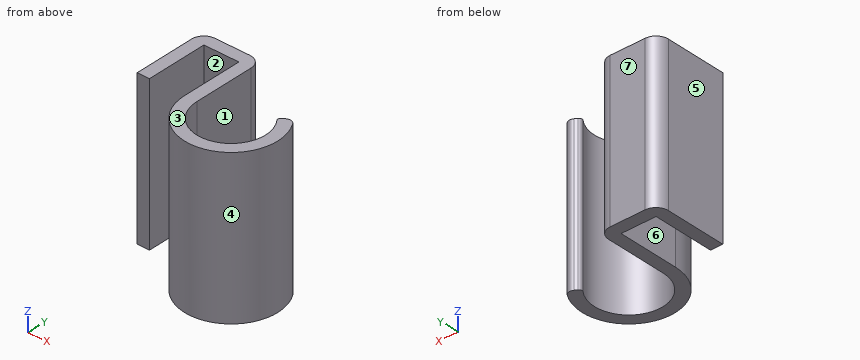
```python
from build123d import *

# Parameters (mm, degrees)
F1_DEPTH = 25
F2_R     = 2
F3_R     = 2
F4_R     = 1
F5_R     = 0.5


with BuildPart() as f1:
    # F0 (on Top) → F1 (new body)
    with BuildSketch(Plane.XY):
        with BuildLine():
            Line((7.7, 12), (-2, 12))
            Line((-2, 12), (-2, 0))
            Line((-2, 0), (0, 0))
            Line((0, 0), (0, 10))
            Line((0, 10), (5.7, 10))
            Line((5.7, 10), (5.7, 0))
            ThreePointArc((5.7, 0), (15.867507, -7.153175), (19.165239, 4.833112))
            Line((19.165239, 4.833112), (17.410544, 3.803082))
            ThreePointArc((17.410544, 3.803082), (15.342175, -5.214357), (7.7, 0))
            Line((7.7, 0), (7.7, 12))
        make_face()
    extrude(amount=F1_DEPTH)

    # F2
    f2_edges = [f1.edges().sort_by_distance(p)[0] for p in [
        (7.7, 12, 12.5),
    ]]
    fillet(f2_edges, radius=F2_R)

    # F3
    f3_edges = [f1.edges().sort_by_distance(p)[0] for p in [
        (-2, 12, 12.5),
    ]]
    fillet(f3_edges, radius=F3_R)

    # F4
    f4_edges = [f1.edges().sort_by_distance(p)[0] for p in [
        (19.165239, 4.833112, 12.5),
    ]]
    fillet(f4_edges, radius=F4_R)

    # F5
    f5_edges = [f1.edges().sort_by_distance(p)[0] for p in [
        (17.410544, 3.803082, 12.5),
    ]]
    fillet(f5_edges, radius=F5_R)


solid = f1.part
```
Here's how the part is built. I have some questions about the finished solid (model axes, mm). Face numbers are marked on the shaded views. A direction names the side the tool comes from. Coordinates: 2 decimals unless noted, no trailing zeros. Loops run counter-clockwise (first coordinate to the right, second up) from the corner with the lowest first, then second, coordinate; pieces in that order, holes last. Notation, with made-up numbers: (26, -24) - (36, -24) arc R13 cw to (36, -11) - close; hole circle Ø5 at (40.5, -25.75). An arc over 180 degrees is marked (long way). Return JSON: item names as keys, results as strings. Group by question number.
Item 1: If we section it at C-C on x = 13.3: Write out the boundary of the cut face in (y, z), and give its area (3 significant figures).
Item 2: If we section it at A-A on y = 6.25: Write out the boundary of the cut face in (x, z), and give its area (3 significant figures).
Item 3: On a 3-axis mill with a long thin cutter (end or side, diameter ignored), from which of +Z, -Z, +X, -X, +Y, -Y can I reach the whole of each face in a straight line? I mean the marked faces 1, 2 and 3. Say none if no direction works.
Item 4: We'd pull the mould along X, two halves only. Please class the marked faces 4, 5, 6 and 7: +X half, -X half, draft (parallel to the pull), parting line (faces both ways), or undercut.
Item 5: Will these pins go through, and if not, where does the flat tip stop? P1, Ø1.5, axis at x = 3, y = 7.5, coming from the -Z side; P2, Ø6, axis at y = -3.5, z = 16, coming from the -X side; P3, Ø1.6, axis at x = -0.5, z = 15.5, coming from the -Y side; P4, Ø1, axis at y = -3.5, z = 20, coming from the +X side.
Item 6: If we section it at B-B on z = 13.25: Write out the boundary of the cut face in (x, y).
Item 7: If we section it at D-D on x = 6.75: Write out the boundary of the cut face in (y, z).
Item 8: I need wall thicknesses on line 1 (X direction, y = 5.25, z = 10); line 2 (X direction, y = -0.25, z = 19.75); line 3 (Y direction, x = 17.75, z = 13.5). Which ranges of each line are inside material? Lowest first, please. Write a range as from..to.
Calculated:
{
 "1": {"outline": "(-7.6, 0) - (-5.6, 0) - (-5.6, 25) - (-7.6, 25) - close", "area": "50.0 mm^2"},
 "2": {"outline": "(-2, 0) - (0, 0) - (0, 25) - (-2, 25) - close; (5.7, 0) - (7.7, 0) - (7.7, 25) - (5.7, 25) - close", "area": "100 mm^2"},
 "3": {"face 1": "+Z, -Z, +Y", "face 2": "+Z, -Z, -Y", "face 3": "+Z, +X, -X, +Y, -Y"},
 "4": {"face 4": "parting line", "face 5": "-X half", "face 6": "undercut", "face 7": "draft"},
 "5": {"P1": "passes through", "P2": "stops at x = 5.72", "P3": "stops at y = 0", "P4": "stops at x = 20.28"},
 "6": {"outline": "(-2, 0) - (0, 0) - (0, 10) - (5.7, 10) - (5.7, 0) arc R7.6 ccw (long way) to (19.74, 4.04) arc R1 ccw to (18.38, 4.37) - (17.92, 4.1) arc R0.5 ccw to (17.77, 3.37) arc R5.6 cw (long way) to (7.7, 0) - (7.7, 10) arc R2 ccw to (5.7, 12) - (0, 12) arc R2 ccw to (-2, 10) - close"},
 "7": {"outline": "(-3.85, 0) - (11.7, 0) - (11.7, 25) - (-3.85, 25) - close"},
 "8": {"line 1": "x = -2..0, 5.7..7.7", "line 2": "x = 5.7..7.71, 18.89..20.9", "line 3": "y = -6.16..-3.4, 3.4..3.94"}
}
